Verification items for the finished model (mm, model axes). A direction names the side the tool comes from. Round coordinates to 2 decimals unless told otherwise and drop trailing zeros. Order: outer loops, then holes, each group sorted by start corner. A loop starts at its lowest first (then second) coordinate and runs counter-clockwise, first axis right, second up. Notation, with made-up numbers: (10, -23.5) -> (38, -23.5) arc R30 cw to (38, 8.5) -> close; hole circle Ø5 at (78, 41). An arc over 180 degrees is marked (long way). Return JSON: item names as keys, results as strings. Group by question number.
Item 1: Scan lines: probe 1 along X at (y, z) = (8.4, 30); probe 2 along Z at (x, y) = (26, 11); probe 3 along Z at (x, y) = (-10, 11.25). Record each from-to range of solid material in increasing order. Write a range as from..to.
Item 2: Sectioned sample at A-A on x = -14.5. Record the cut outline in (y, z).
Item 3: Sectioned sample at D-D on y = 2.75. Record the cut outline in (x, z), plus the area to 3 significant figures.
Item 4: Draft check along Z on faces 1 (the flat face through (26, 11, -25.1)), 2 (the flat face through (32.5, 6, 1)). Enter one of: pulls with the +Z half, pulls with the -Z half, needs draft (parallel to the pull), parting line crosses it, or undercut.
Item 5: Sectioned sample at B-B on z = 30. Record the cut outline in (x, y).
Item 6: Depth check by flat-ended pin: pin 1 Ø4.5 at (x, z) = (-14.5, -30) entering from +Y; pin 2 Ø2 at (y, z) = (3, -2) entering from +X; pin 3 Ø1.5 at (x, z) = (9, -10) entering from -Y. Enter the tip coordinate at first touch or a pass-through.
Item 7: Access from +Z, -Z, +X, -X, +Y, -Y to the whole of each face (thin tool, end or side, straight path). Record for faces 3 (the cylindrical face through (-13.899, 8.521, 31.908)), 4 (the flat face through (-3, 0, -33)), 5 (the flat face through (-29.1, 11, 30)), 6 (the flat face through (0, 7, 0)), 7 (the flat face through (31, 1.399, 0)).
Item 8: Sectioned sample at C-C on x = -25.5. Record the cut outline in (y, z).
```python
from build123d import *

# Parameters (mm, degrees)
SKETCH1_W           = 65
SKETCH1_H           = 80
BOSS_EXTRUDE1_DEPTH = 12
SKETCH3_W           = 58.2
SKETCH3_H           = 65
CUT_EXTRUDE4_DEPTH  = 2
SKETCH6_R           = 2
CUT_EXTRUDE5_DEPTH  = 10
SKETCH7_W           = 58.2
SKETCH7_H           = 65
CUT_EXTRUDE6_DEPTH  = 7
CUT_EXTRUDE8_DEPTH  = 6
SKETCH11_W          = 3
SKETCH11_H          = 2
BOSS_EXTRUDE3_DEPTH = 6
SKETCH13_W          = 3
SKETCH13_H          = 2
BOSS_EXTRUDE4_DEPTH = 6


with BuildPart() as part:
    # Sketch1 → Boss-Extrude1 (new body)
    with BuildSketch(Plane(origin=(0, 0, 0), x_dir=(1, 0, 0), z_dir=(0, 1, 0))):
        Rectangle(SKETCH1_W, SKETCH1_H)
    extrude(amount=BOSS_EXTRUDE1_DEPTH)

    # Sketch3 → Cut-Extrude4 (cut)
    with BuildSketch(Plane(origin=(0, 12, 0), x_dir=(1, 0, 0), z_dir=(0, 1, 0))):
        Rectangle(SKETCH3_W, SKETCH3_H)
    extrude(amount=-CUT_EXTRUDE4_DEPTH, mode=Mode.SUBTRACT)

    # Sketch6 → Cut-Extrude5 (cut)
    with BuildSketch(Plane(origin=(0, 10, 0), x_dir=(1, 0, 0), z_dir=(0, 1, 0))):
        with Locations(Location((14.5, 30, 0), (0, 0, 270))):  # turned: the seam where the file's is
            Circle(SKETCH6_R)
        with Locations(Location((-14.5, 30, 0), (0, 0, 90))):  # turned: the seam where the file's is
            Circle(SKETCH6_R)
        with Locations(Location((-14.5, -30, 0), (0, 0, 270))):  # turned: the seam where the file's is
            Circle(SKETCH6_R)
        with Locations(Location((14.5, -30, 0), (0, 0, 90))):  # turned: the seam where the file's is
            Circle(SKETCH6_R)
    extrude(amount=-CUT_EXTRUDE5_DEPTH, mode=Mode.SUBTRACT)

    # Sketch7 → Cut-Extrude6 (cut)
    with BuildSketch(Plane(origin=(0, 0, 0), x_dir=(1, 0, 0), z_dir=(0, 1, 0))):
        Rectangle(SKETCH7_W, SKETCH7_H)
    extrude(amount=CUT_EXTRUDE6_DEPTH, mode=Mode.SUBTRACT)

    # Sketch10 → Cut-Extrude8 (cut)
    with BuildSketch(Plane.ZY.offset(-29.1)):
        with BuildLine():
            Line((-2.277690302, 5.601430768), (2.277690302, 5.601430768))
            ThreePointArc((2.277690302, 5.601430768), (4.379121071, 3.5), (2.277690302, 1.398569232))
            Line((2.277690302, 1.398569232), (-2.277690302, 1.398569232))
            ThreePointArc((-2.277690302, 1.398569232), (-4.379121071, 3.5), (-2.277690302, 5.601430768))
        make_face()
    extrude(amount=-CUT_EXTRUDE8_DEPTH, mode=Mode.SUBTRACT)

    # Sketch11 → Boss-Extrude3 (add)
    with BuildSketch(Plane.ZY.offset(-29.1)):
        with Locations((-26.6, 11)):
            Rectangle(SKETCH11_W, SKETCH11_H)
        with Locations((26.6, 11)):
            Rectangle(SKETCH11_W, SKETCH11_H)
    extrude(amount=BOSS_EXTRUDE3_DEPTH)

    # Sketch13 → Boss-Extrude4 (add)
    with BuildSketch(Plane(origin=(-29.1, 0, 0), x_dir=(0, 0, -1), z_dir=(1, 0, 0))):
        with Locations((26.6, 11)):
            Rectangle(SKETCH13_W, SKETCH13_H)
        with Locations((-26.6, 11)):
            Rectangle(SKETCH13_W, SKETCH13_H)
    extrude(amount=BOSS_EXTRUDE4_DEPTH)


solid = part.part
```
Recorded:
{
 "1": {"probe 1": "-32.5..-16.5, -12.5..12.5, 16.5..32.5", "probe 2": "-40..-32.5, -28.1..-25.1, 25.1..28.1, 32.5..40", "probe 3": "-40..-32.5, 32.5..40"},
 "2": {"outline": "(0, -40) -> (12, -40) -> (12, -32.5) -> (10, -32.5) -> (10, -32) -> (7, -32) -> (7, -32.5) -> (0, -32.5) -> close; (0, 32.5) -> (7, 32.5) -> (7, 32) -> (10, 32) -> (10, 32.5) -> (12, 32.5) -> (12, 40) -> (0, 40) -> close; (7, -28) -> (10, -28) -> (10, 28) -> (7, 28) -> close"},
 "3": {"outline": "(-32.5, -40) -> (32.5, -40) -> (32.5, -4.24) -> (29.1, -4.24) -> (29.1, -32.5) -> (-29.1, -32.5) -> (-29.1, 32.5) -> (29.1, 32.5) -> (29.1, 4.24) -> (32.5, 4.24) -> (32.5, 40) -> (-32.5, 40) -> close", "area": "1,390 mm²"},
 "4": {"face 1": "undercut", "face 2": "needs draft"},
 "5": {"outline": "(-32.5, 0) -> (-29.1, 0) -> (-29.1, 7) -> (-16.5, 7) -> (-16.5, 10) -> (-29.1, 10) -> (-29.1, 12) -> (-32.5, 12) -> close; (-12.5, 7) -> (12.5, 7) -> (12.5, 10) -> (-12.5, 10) -> close; (16.5, 7) -> (29.1, 7) -> (29.1, 0) -> (32.5, 0) -> (32.5, 12) -> (29.1, 12) -> (29.1, 10) -> (16.5, 10) -> close"},
 "6": {"pin 1": "y = 10", "pin 2": "x = -29.1", "pin 3": "y = 7"},
 "7": {"face 3": "+Y, -Y", "face 4": "+Z, -Z, +X, -X, -Y", "face 5": "+Y", "face 6": "-Y", "face 7": "+X"},
 "8": {"outline": "(0, -40) -> (12, -40) -> (12, -32.5) -> (10, -32.5) -> (10, -28.1) -> (12, -28.1) -> (12, -25.1) -> (10, -25.1) -> (10, 25.1) -> (12, 25.1) -> (12, 28.1) -> (10, 28.1) -> (10, 32.5) -> (12, 32.5) -> (12, 40) -> (0, 40) -> (0, 32.5) -> (7, 32.5) -> (7, -32.5) -> (0, -32.5) -> close"}
}
